from build123d import *

# Parameters (mm, degrees)
SKETCH1_W           = 60
SKETCH1_H           = 15
BOSS_EXTRUDE1_DEPTH = 3
SKETCH2_W           = 15
SKETCH2_H           = 50
BOSS_EXTRUDE2_DEPTH = 3
SKETCH3_W           = 5
SKETCH3_H           = 5
BOSS_EXTRUDE3_DEPTH = 15
SKETCH4_R           = 1.5
CUT_EXTRUDE1_DEPTH  = 80.529868603
FILLET1_R           = 2
SKETCH5_W           = 15
SKETCH5_H           = 15
CUT_EXTRUDE2_DEPTH  = 2.5
SKETCH6_R           = 2
BOSS_EXTRUDE4_DEPTH = 15
SKETCH7_R           = 1.5
CUT_EXTRUDE3_DEPTH  = 82.049367672
SKETCH8_W           = 10
SKETCH8_H           = 4.50152391
CUT_EXTRUDE4_DEPTH  = 2.5
SKETCH11_W          = 4.242640687
SKETCH11_H          = 15
BOSS_EXTRUDE5_DEPTH = 50


with BuildPart() as part:
    # Sketch1 → Boss-Extrude1 (new body)
    with BuildSketch(Plane(origin=(0, 0, 0), x_dir=(1, 0, 0), z_dir=(0, 1, 0))):
        with Locations((30, 7.5)):
            Rectangle(SKETCH1_W, SKETCH1_H)
    extrude(amount=BOSS_EXTRUDE1_DEPTH)

    # Sketch2 → Boss-Extrude2 (add)
    with BuildSketch(Plane.ZY):
        with Locations((-7.5, 25)):
            Rectangle(SKETCH2_W, SKETCH2_H)
    extrude(amount=BOSS_EXTRUDE2_DEPTH)

    # Sketch3 → Boss-Extrude3 (add)
    with BuildSketch(Plane(origin=(0, 0, -15), x_dir=(-1, 0, 0), z_dir=(0, 0, -1))):
        with Locations((0.5, 2.5)):
            Rectangle(SKETCH3_W, SKETCH3_H)
    extrude(amount=-BOSS_EXTRUDE3_DEPTH)

    # Sketch4 → Cut-Extrude1 (cut, through all)
    with BuildSketch(Plane(origin=(0, 0, -15), x_dir=(-1, 0, 0), z_dir=(0, 0, -1))):
        with Locations((0.5, 2.5)):
            Circle(SKETCH4_R)
    extrude(amount=-CUT_EXTRUDE1_DEPTH, mode=Mode.SUBTRACT)

    # Fillet1
    fillet1_edges = [part.edges().sort_by_distance(p)[0] for p in [
        (-3, 0, -7.5),
    ]]
    fillet(fillet1_edges, radius=FILLET1_R)

    # Sketch5 → Cut-Extrude2 (cut)
    with BuildSketch(Plane(origin=(0, 0, -15), x_dir=(-1, 0, 0), z_dir=(0, 0, -1))):
        with Locations((-4.5, 7.5)):
            Rectangle(SKETCH5_W, SKETCH5_H)
    cut_extrude2 = extrude(amount=-CUT_EXTRUDE2_DEPTH, mode=Mode.SUBTRACT)

    # Mirror1: Cut-Extrude2 across plane
    add(cut_extrude2.mirror(Plane(origin=(0, 0, -7.5), x_dir=(1, 0, 0), z_dir=(0, 0, -1))), mode=Mode.SUBTRACT)

    # Sketch6 → Boss-Extrude4 (add)
    with BuildSketch(Plane(origin=(0, 0, -15), x_dir=(-1, 0, 0), z_dir=(0, 0, -1))):
        with Locations((-60, 1.5)):
            Circle(SKETCH6_R)
    extrude(amount=-BOSS_EXTRUDE4_DEPTH)

    # Sketch7 → Cut-Extrude3 (cut, through all)
    with BuildSketch(Plane(origin=(0, 0, -15), x_dir=(-1, 0, 0), z_dir=(0, 0, -1))):
        with Locations((-60, 1.5)):
            Circle(SKETCH7_R)
    extrude(amount=-CUT_EXTRUDE3_DEPTH, mode=Mode.SUBTRACT)

    # Sketch8 → Cut-Extrude4 (cut)
    with BuildSketch(Plane(origin=(0, 0, -15), x_dir=(-1, 0, 0), z_dir=(0, 0, -1))):
        with Locations((-57, 1.249238045)):
            Rectangle(SKETCH8_W, SKETCH8_H)
    cut_extrude4 = extrude(amount=-CUT_EXTRUDE4_DEPTH, mode=Mode.SUBTRACT)

    # Mirror2: Cut-Extrude4 across plane
    add(cut_extrude4.mirror(Plane(origin=(0, 0, -7.5), x_dir=(1, 0, 0), z_dir=(0, 0, -1))), mode=Mode.SUBTRACT)

    # Sketch11 → Boss-Extrude5 (add)
    with BuildSketch(Plane(origin=(23.5, 23.5, 0), x_dir=(0.7071067811865476, -0.7071067811865476, 0), z_dir=(0.7071067811865476, 0.7071067811865476, 0))):
        with Locations((-35.355339059, 7.5)):
            Rectangle(SKETCH11_W, SKETCH11_H)
    extrude(amount=BOSS_EXTRUDE5_DEPTH)


solid = part.part
Could you check a few things on this model? Use its own coordinates, in mm. A direction names the side the tool comes from. Round coordinates to 2 decimals unless told otherwise and drop trailing zeros. Write each loop counter-clockwise with the first axis right and the second up, starting at its lowest first coordinate (ties: lowest second). Pieces come first, ordered by that corner, then holes. Notation, with made-up numbers: (14, -32) - (58, -32) arc R31 ccw to (58, -7) - close; hole circle Ø4 at (65, -24). An arc over 180 degrees is marked (long way). Put each result on its own line as item: value. Start each with the question number.
(1) I want a section at A-A, the plane x = 60. Please give me the cut outline in (y, z), plus the area to 3 significant figures.
(2) I want a section at D-D, the plane y = 29. Please give me the cut outline in (x, z), plus the area to 3 significant figures.
(3) For faces 1 (the flat face through (29, 0, -8)), 2 (the flat face through (-1, 15, -1)), 3 (the flat face through (17, 64, -7)), 4 (the flat face through (12, 1, -14)), which set-ups out of +Z, -Z, +X, -X, +Y, -Y let a thin tool reach every point of the face, with its end or its side?
(4) Will these pins go through, and if not, where does the flat tip stop? pin 1 (3 mm diameter, centred on y = 26.5, z = -3, fed in from +X); pin 2 (12 mm diameter, centred on x = 4, y = 4.5, fed in from -Z); pin 3 (0.6 mm diameter, centred on y = 3.5, z = -10, fed in from +X).
(5) I want a section at B-B, the plane z = -3.5. Please give me the cut outline in (x, y), plus the area to 3 significant figures.
(6) Thinking about a two-plate mould opening in X: for faces 5 (the flat face through (-3, 26, -8)), 6 (the flat face through (30, 3, -8)), 7 (the flat face through (-1, 15, -14)), 8 (the flat face through (52, 1, -1)), which applies, released by +X, released by -X, zero draft, split by the parting line, or undercut?
(7) I want a section at C-C, the plane x = 28. Please give me the cut outline in (y, z), plus the area to 3 significant figures.
(8) I need wall thicknesses on probe 1 along Y at (x, z) = (60, -7.25); probe 2 along X at (y, z) = (34, -8.75); probe 3 along Y at (x, z) = (45, -11.25). Which ranges of each line are inside material? Lowest first, please.
Here are the results:
1. outline: (-0.5, -12.5) - (0, -12.5) - (0, -2.5) - (-0.5, -2.5) - close; (3, -12.5) - (3.5, -12.5) - (3.5, -2.5) - (3, -2.5) - close
1. area: 10.0 mm^2
2. outline: (-3, -15) - (0, -15) - (0, 0) - (-3, 0) - close
2. area: 45.0 mm^2
3. face 1: +Z, -Z, -X, -Y
3. face 2: +Z, +X, -X, -Y
3. face 3: +Z, -Z, +X
3. face 4: -Z, -X, -Y
4. pin 1: stops at x = 0
4. pin 2: stops at z = -12.5
4. pin 3: stops at x = 61.05
5. outline: (-3, 2) arc R2 ccw to (-1, 0) - (58.68, 0) arc R2 ccw (long way) to (58.68, 3) - (2, 3) - (2, 5) - (0, 5) - (0, 47) - (35.36, 82.36) - (32.36, 85.36) - (-3, 50) - close; hole circle Ø3 at (-0.5, 2.5); hole circle Ø3 at (60, 1.5)
5. area: 534 mm^2
6. face 5: released by -X
6. face 6: undercut
6. face 7: zero draft
6. face 8: released by +X
7. outline: (0, -15) - (3, -15) - (3, 0) - (0, 0) - close; (75, -15) - (81, -15) - (81, 0) - (75, 0) - close
7. area: 135 mm^2
8. probe 1: y = -0.5 to 0, 3 to 3.5
8. probe 2: x = -3 to 0
8. probe 3: y = 0 to 3
